Could you check a few things on this drawing? It's one solid part, dimensions in mm from its lowest x, y, z. A direction names the side the tool comes from. Give positions to 0.01 mm unless a question says otherwise; leave off trailing zeros. Loops run counter-clockwise (first coordinate to the right, second up) from the corner with the lowest first, then second, coordinate; pieces in that order, holes last. Notation, with made-up numbers: M 63,85 L 68,85 A23 ccw 68,112 Z; hole C 60,5.25 d8. An arc over 180 degrees is marked long. Return JSON: item names as keys, results as strings. Group by question number.
1. If we section it at A-A (z = 10): Write out the boundary of the cut face in (x, y).
2. If we mould it in two halves opening along X, with no side actions, what happens to the marked faces 1, 2, 3 and 4? For each: +X half, -X half, draft (parallel to the pull), parting line (faces both ways), or undercut.
3. If we section it at D-D (z = 29): Write out the boundary of the cut face in (x, y).
4. Please list where these lines run through material, in increasing order: line 1 (Z direction, x = 55, y = 1.2); line 2 (X direction, y = 1.5, z = 25); line 3 (X direction, y = 2.5, z = 26).
5. If we section it at B-B (x = 55): Write out the boundary of the cut face in (y, z).
6. If we section it at C-C (y = 21.75): Write out the boundary of the cut face in (x, z).
7. For pin 1 (6.5 mm diameter, centred on x = 55, z = 25, fed in from +Y); pin 2 (1 mm diameter, centred on y = 18, z = 7.5, fed in from -X); pin 3 (10 mm diameter, centred on y = 17.5, z = 26, fed in from +X), each with a flat end and sliding along its axis, tell me the tip position at first contact or that it passes through.
8. For the marked faces 5, 6 and 7, which set-ups out of +Z, -Z, +X, -X, +Y, -Y let a thin tool reach every point of the face, with its end or its side?
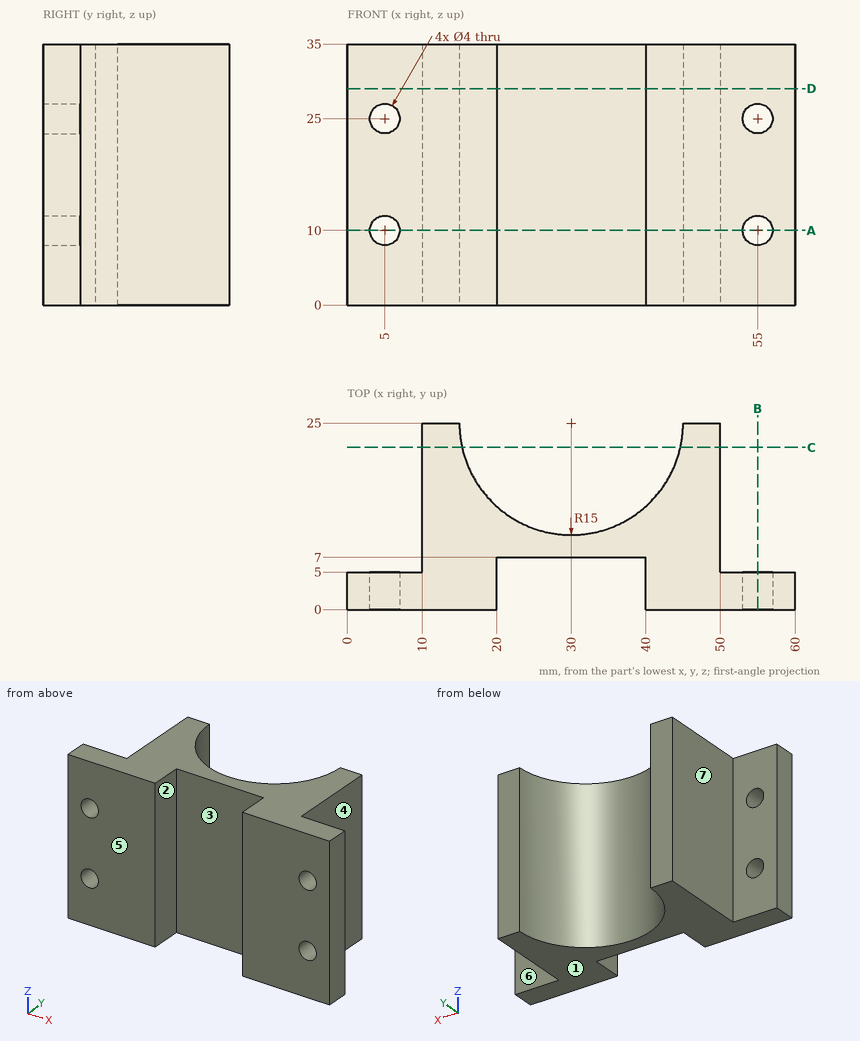
Answer:
{
 "1": {"outline": "M 0,0 L 3,0 L 3,5 L 0,5 Z; M 7,0 L 20,0 L 20,7 L 40,7 L 40,0 L 53,0 L 53,5 L 50,5 L 50,25 L 45,25 A15 cw 15,25 L 10,25 L 10,5 L 7,5 Z; M 57,0 L 60,0 L 60,5 L 57,5 Z"},
 "2": {"face 1": "draft", "face 2": "undercut", "face 3": "undercut", "face 4": "+X half"},
 "3": {"outline": "M 0,0 L 20,0 L 20,7 L 40,7 L 40,0 L 60,0 L 60,5 L 50,5 L 50,25 L 45,25 A15 cw 15,25 L 10,25 L 10,5 L 0,5 Z"},
 "4": {"line 1": "z = 0 to 8, 12 to 23, 27 to 35", "line 2": "x = 0 to 3, 7 to 20, 40 to 53, 57 to 60", "line 3": "x = 0 to 3.27, 6.73 to 20, 40 to 53.27, 56.73 to 60"},
 "5": {"outline": "M 0,0 L 5,0 L 5,8 L 0,8 Z; M 0,12 L 5,12 L 5,23 L 0,23 Z; M 0,27 L 5,27 L 5,35 L 0,35 Z"},
 "6": {"outline": "M 10,0 L 15.36,0 L 15.36,35 L 10,35 Z; M 44.64,0 L 50,0 L 50,35 L 44.64,35 Z"},
 "7": {"pin 1": "stops at y = 5", "pin 2": "stops at x = 10", "pin 3": "stops at x = 50"},
 "8": {"face 5": "+Z, -Z, +X, -X, -Y", "face 6": "+Z, -Z, +X, +Y", "face 7": "+Z, -Z, -X, +Y"}
}
